The listing builds one solid part. Answer for the finished solid, in the listing's coordinates (mm). A direction names the side the tool comes from. Give positions to 0.01 mm unless a question says otherwise; leave off trailing zeros. Write each loop counter-clockwise with the first axis right and the second up, starting at its lowest first coordinate (ties: lowest second). Pieces come first, ordered by that corner, then holes. Notation, with made-up numbers: (37.5, -4.75) - (96.5, -4.75) arc R34 ccw to (96.5, 34.25) - close; hole circle Ø9 at (78.25, 77.5). An arc over 180 degrees is marked (long way). Use a Markdown table: item, result. Add a question column.
from build123d import *

# Parameters (mm, degrees)
BOSS_EXTRUDE1_DEPTH     = 8
SKETCH2_R               = 3.15
CUT_EXTRUDE1_DEPTH      = 8
SKETCH3_W               = 9.706264803
SKETCH3_H               = 21
SKETCH3_R               = 2.15
BOSS_EXTRUDE3_DEPTH     = 2
SKETCH4_W               = 42
SKETCH4_H               = 23
CUT_EXTRUDE4_DEPTH      = 16
CUT_EXTRUDE4_DEPTH_BACK = 16
CUT_EXTRUDE5_DEPTH      = 2.5
SKETCH8_R               = 2.15
CUT_EXTRUDE8_DEPTH      = 21.6
SKETCH9_R               = 4
CUT_EXTRUDE9_DEPTH      = 2.6
FILLET2_R               = 0.5


with BuildPart() as part:
    # Sketch1 → Boss-Extrude1 (new body)
    with BuildSketch(Plane(origin=(0, 0, 0), x_dir=(1, 0, 0), z_dir=(0, 1, 0))):
        with BuildLine():
            ThreePointArc((10.980762114, 15), (15.374160396, 4.393398282), (25.980762114, 0))
            Line((25.980762114, 0), (65.009618943, 0))
            ThreePointArc((65.009618943, 0), (71.630509288, 1.991812799), (76.05347061, 7.306031492))
            Line((76.05347061, 7.306031492), (90.667824887, 41.690318597))
            Line((90.667824887, 41.690318597), (92.106342015, 45.074825706))
            Line((92.106342015, 45.074825706), (94.659597169, 51.082060554))
            ThreePointArc((94.659597169, 51.082060554), (93.365016587, 65.225634119), (80.854782585, 71.949521188))
            Line((80.854782585, 71.949521188), (30.067550518, 71.949521188))
            ThreePointArc((30.067550518, 71.949521188), (19.979275987, 68.05027418), (15.13589136, 58.37975012))
            Line((15.13589136, 58.37975012), (14.014444666, 46.671792448))
            Line((14.014444666, 46.671792448), (10.980762114, 15))
        make_face()
    extrude(amount=BOSS_EXTRUDE1_DEPTH)

    # Sketch2 → Cut-Extrude1 (cut)
    with BuildSketch(Plane(origin=(0, 8, 0), x_dir=(1, 0, 0), z_dir=(0, 1, 0))):
        with Locations((30, 10)):
            Circle(SKETCH2_R)
        with Locations((60, 10)):
            Circle(SKETCH2_R)
    extrude(amount=-CUT_EXTRUDE1_DEPTH, mode=Mode.SUBTRACT)

    # Sketch3 → Boss-Extrude3 (add)
    with BuildSketch(Plane(origin=(0, 8, 0), x_dir=(1, 0, 0), z_dir=(0, 1, 0))):
        with Locations((30.236867599, 54.358166274)):
            Rectangle(SKETCH3_W, SKETCH3_H)
        with Locations((30.81, 49.608166274)):
            Circle(SKETCH3_R, mode=Mode.SUBTRACT)
        with Locations((30.81, 59.108166274)):
            Circle(SKETCH3_R, mode=Mode.SUBTRACT)
        Polygon((75.15, 43.858166274), (85.15, 43.858166274), (85.15, 62.709957967), (85.15, 64.858166274), (75.15, 64.858166274), (75.11, 54.358166274), align=None)
        with Locations((79.81, 49.608166274)):
            Circle(SKETCH3_R, mode=Mode.SUBTRACT)
        with Locations((79.81, 59.108166274)):
            Circle(SKETCH3_R, mode=Mode.SUBTRACT)
    extrude(amount=BOSS_EXTRUDE3_DEPTH)

    # Sketch4 → Cut-Extrude4 (cut, two sides)
    with BuildSketch(Plane(origin=(0, 8, 0), x_dir=(1, 0, 0), z_dir=(0, 1, 0))) as cut_extrude4_sk:
        with Locations((55.09, 54.358166274)):
            Rectangle(SKETCH4_W, SKETCH4_H)
    extrude(amount=CUT_EXTRUDE4_DEPTH, mode=Mode.SUBTRACT)
    extrude(cut_extrude4_sk.sketch, amount=-CUT_EXTRUDE4_DEPTH_BACK, mode=Mode.SUBTRACT)

    # Sketch5 → Cut-Extrude5 (cut)
    with BuildSketch(Plane(origin=(0, 10, 0), x_dir=(1, 0, 0), z_dir=(0, 1, 0))):
        Polygon((76.09, 54.358166274), (76.09, 55.358166274), (82.59, 55.358166274), (82.59, 53.358166274), (76.09, 53.358166274), align=None)
        Polygon((27.59, 54.358166274), (27.59, 55.358166274), (34.09, 55.358166274), (34.09, 53.358166274), (27.59, 53.358166274), align=None)
    extrude(amount=-CUT_EXTRUDE5_DEPTH, mode=Mode.SUBTRACT)

    # Sketch8 → Cut-Extrude8 (cut)
    with BuildSketch(Plane(origin=(0, 8, 0), x_dir=(1, 0, 0), z_dir=(0, 1, 0))):
        with Locations((30.81, 49.608166274)):
            Circle(SKETCH8_R)
        with Locations((30.81, 59.108166274)):
            Circle(SKETCH8_R)
        with Locations((79.81, 59.108166274)):
            Circle(SKETCH8_R)
        with Locations((79.81, 49.608166274)):
            Circle(SKETCH8_R)
    extrude(amount=-CUT_EXTRUDE8_DEPTH, mode=Mode.SUBTRACT)

    # Sketch9 → Cut-Extrude9 (cut)
    with BuildSketch(Plane.XZ):
        with Locations((30.81, -59.108166274)):
            Circle(SKETCH9_R)
        with Locations((30.81, -49.608166274)):
            Circle(SKETCH9_R)
        with Locations((79.81, -59.108166274)):
            Circle(SKETCH9_R)
        with Locations((79.81, -49.608166274)):
            Circle(SKETCH9_R)
    extrude(amount=-CUT_EXTRUDE9_DEPTH, mode=Mode.SUBTRACT)

    # Fillet2
    fillet2_edges = [part.edges().sort_by_distance(p)[0] for p in [
        (76.09, 1.3, -51.07840435),
        (76.09, 1.3, -48.137928198),
        (76.09, 1.3, -60.57840435),
        (76.09, 1.3, -57.637928198),
        (34.09, 1.3, -56.818712191),
        (34.09, 1.3, -61.397620358),
        (34.09, 1.3, -47.318712191),
        (34.09, 1.3, -51.897620358),
    ]]
    fillet(fillet2_edges, radius=FILLET2_R)


solid = part.part
1. The part is cut by section A-A (x = 50). Give the vertices of the cut face in (y, z), and give its area (3 significant figures).
2. Consider L1, parallel to Z at x = 30.81, y = 8.7; L2, parallel to Z at x = 79.81, y = 6.1; L3, parallel to Z at x = 79.81, y = 0.7. Determine where each line is inside the solid, lowest interval first. Write a range as [from, to].
3. The part is cut by section D-D (z = -10). Give the vertices of the cut face in (x, y), and give its area (3 significant figures).
4. The part is cut by section C-C (y = 9). Give the vertices of the cut face in (x, z).
5. The part is cut by section B-B (x = 60). Give the vertices of the cut face in (y, z), and give its area (3 significant figures).
6. Given P1, Ø4, axis at x = 30.81, z = -59.11, coming from the -Y side; P2, Ø1, axis at x = 41.5, z = -22.5, coming from the +Y side; P3, Ø6, axis at x = 31, z = -59.5, coming from the -Y side; P4, Ø10.5, axis at x = 30.81, z = -49.61, coming from the +Y side, each flat-ended and moving along its own axis, determine where each tip first touches the part or whether it passes through.
7. For a pull along Z with two mould halves and no side action, classify faces 6 (the cylindrical face through (93.48, 3.94, -65.05)), 7 (the flat face through (78.2, 2.6, -51.3)), 8 (the flat face through (43, 8, -36)) as released by +Z, released by -Z, zero draft, split by the parting line, or undercut.
8. Which of the six approach directions +Z, -Z, +X, -X, +Y, -Y give full straight-line access (tool end or side, diameter ignored) to faces 1 (the flat face through (30, 9, -64.858)), 2 (the flat face through (31, 9, -53.358)), 3 (the flat face through (55, 4, -65.858)), 4 (the flat face through (32, 2.6, -57)), 5 (the flat face through (30, 9, -43.858))?
Check values:
| question | item | result |
|---|---|---|
| 1 | outline | (0, -71.95) - (8, -71.95) - (8, -65.86) - (0, -65.86) - close; (0, -42.86) - (8, -42.86) - (8, 0) - (0, 0) - close |
| 1 | area | 392 mm2 |
| 2 | L1 | z = [-64.86, -61.26], [-56.96, -55.36], [-53.36, -51.76], [-47.46, -43.86] |
| 2 | L2 | z = [-71.95, -61.26], [-56.96, -51.76], [-47.46, -16.14] |
| 2 | L3 | z = [-71.95, -63.11], [-55.11, -53.61], [-45.61, -16.14] |
| 3 | outline | (11.84, 0) - (26.85, 0) - (26.85, 8) - (11.84, 8) - close; (33.15, 0) - (56.85, 0) - (56.85, 8) - (33.15, 8) - close; (63.15, 0) - (77.2, 0) - (77.2, 8) - (63.15, 8) - close |
| 3 | area | 422 mm2 |
| 4 | outline | (25.38, -64.86) - (34.09, -64.86) - (34.09, -55.36) - (27.59, -55.36) - (27.59, -53.36) - (34.09, -53.36) - (34.09, -43.86) - (25.38, -43.86) - close; (76.09, -64.86) - (85.15, -64.86) - (85.15, -43.86) - (76.09, -43.86) - (76.09, -53.36) - (82.59, -53.36) - (82.59, -55.36) - (76.09, -55.36) - close; hole circle Ø4.3 at (30.81, -59.11); hole circle Ø4.3 at (30.81, -49.61); hole circle Ø4.3 at (79.81, -59.11); hole circle Ø4.3 at (79.81, -49.61) |
| 5 | outline | (0, -71.95) - (8, -71.95) - (8, -65.86) - (0, -65.86) - close; (0, -42.86) - (8, -42.86) - (8, -13.15) - (0, -13.15) - close; (0, -6.85) - (8, -6.85) - (8, 0) - (0, 0) - close |
| 5 | area | 341 mm2 |
| 6 | P1 | passes through |
| 6 | P2 | stops at y = 8 |
| 6 | P3 | stops at y = 2.6 |
| 6 | P4 | stops at y = 10 |
| 7 | face 6 | split by the parting line |
| 7 | face 7 | undercut |
| 7 | face 8 | zero draft |
| 8 | face 1 | -Z, +X, -X, +Y |
| 8 | face 2 | +Y |
| 8 | face 3 | +Y, -Y |
| 8 | face 4 | -Y |
| 8 | face 5 | +Z, +X, -X, +Y |
